Verification items for this drawing (mm, ordinates from the low corner). Coordinates: 2 decimals unless noted, no trailing zeros. Order: outer loops, then holes, each group sorted by start corner. A loop starts at its lowest first (then second) coordinate and runs counter-clockwise, first axis right, second up. Notation, with made-up numbers: M 48.25,73 L 74.25,73 A28 ccw 74.25,97 Z; hole C -2,-22.5 d6. An arc over 180 degrees is marked long. Write item = value, one per line.
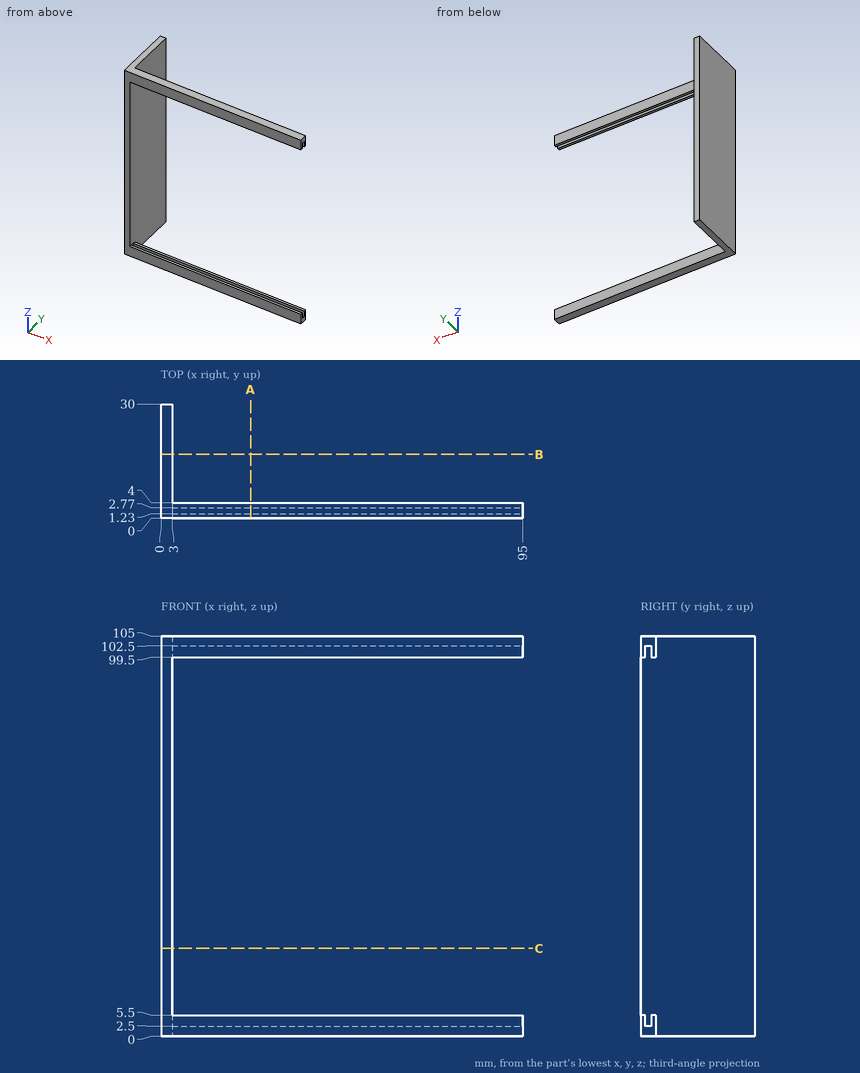
Item 1: Gauge pin test, flat ends, axial feed: pin 1 (3 mm diameter, centred on x = 67, z = 101.5, fed in from +Y); pin 2 (9 mm diameter, centred on y = 17.5, z = 71, fed in from +X). Record the tip position at first contact, or that the pin passes through.
Report:
pin_1 = 4
pin_2 = 3
Item 2: Scan lines: L1, parallel to X at y = 21.75, z = 47; L2, parallel to Z at x = 53, y = 3.75; L3, parallel to Z at x = 26, y = 1.5. Record each from-to range of solid material in increasing order. Write a range as from..to.
Report:
L1 = 0..3
L2 = 0..5.5, 99.5..105
L3 = 0..2.5, 102.5..105
Item 3: Sectioned sample at A-A, the plane x = 23.5. Enter the section's corners in (y, z), then the cut area to 3 significant figures.
Report:
outline = M 0,0 L 4,0 L 4,5.5 L 2.77,5.5 L 2.77,2.5 L 1.23,2.5 L 1.23,5.5 L 0,5.5 Z; M 0,99.5 L 1.23,99.5 L 1.23,102.5 L 2.77,102.5 L 2.77,99.5 L 4,99.5 L 4,105 L 0,105 Z
area = 34.8 mm^2
Item 4: Sectioned sample at C-C, the plane z = 23. Enter the section's corners in (x, y), then the cut area to 3 significant figures.
Report:
outline = M 0,0 L 3,0 L 3,30 L 0,30 Z
area = 90.0 mm^2
Item 5: Sectioned sample at B-B, the plane y = 16.75. Enter the section's corners in (x, z), then the cut area to 3 significant figures.
Report:
outline = M 0,0 L 3,0 L 3,105 L 0,105 Z
area = 315 mm^2
